Input: part model. Units: mm. Frame: model coordinates. Face numbers are marked on the shaded views. Coordinates: 2 decimals unless noted, no trailing zeros. Loops run counter-clockwise (first coordinate to the right, second up) from the corner with the lowest first, then second, coordinate; pieces in that order, holes last.
```python
from build123d import *

# Parameters (mm, degrees)
F0_R          = 6.3
F0_R_2        = 2.5
F1_DEPTH      = 5
F1_DEPTH_BACK = 6
F6_D          = 2.5
F6_DEPTH      = 5
F6_START      = 0.1252531
F6_TIP        = 0.7510757738


with BuildPart() as f1:
    # F0 (on Front) → F1 (new body, two sides)
    with BuildSketch(Plane.XZ) as f1_sk:
        Circle(F0_R)
        Circle(F0_R_2, mode=Mode.SUBTRACT)
    extrude(amount=-F1_DEPTH)
    extrude(f1_sk.sketch, amount=F1_DEPTH_BACK)

    # F2 (on Right) → F3 (revolve, cut)
    with BuildSketch(Plane.YZ):
        with BuildLine():
            ThreePointArc((0, 6.3), (-2.5, 8.8), (-5, 6.3))
            Line((-5, 6.3), (0, 6.3))
        make_face()
        with BuildLine():
            Line((0, 6.3), (-5, 6.3))
            ThreePointArc((-5, 6.3), (-2.5, 3.8), (0, 6.3))
        make_face()
    revolve(axis=Axis((0, -6, 0), (0, -1, 0)), mode=Mode.SUBTRACT)

    # F6
    # its depths count from where the whole tool has entered the part; down to there all is cleared
    with Locations(Plane.YZ.offset(6.3).offset(-F6_START)):
        with Locations((2.5, 0)):
            Hole(F6_D / 2, depth=F6_DEPTH)
            with Locations((0, 0, -(F6_DEPTH + F6_TIP / 2))):  # 118° drill point
                Cone(0, F6_D / 2, F6_TIP, mode=Mode.SUBTRACT)


solid = f1.part
```
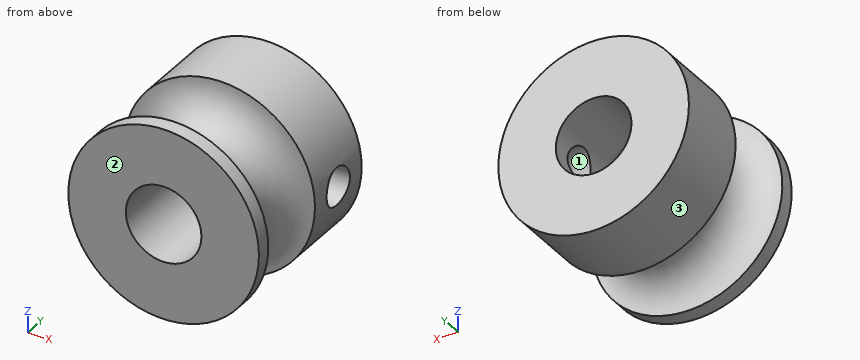
Item 1: Section query A-A (x = 0). Output: boundary loops of the cut face in (y, z), then the cut area to 3 significant figures.
Result:
outline: (-6, -6.3) - (-5, -6.3) arc R2.5 cw to (0, -6.3) - (5, -6.3) - (5, -2.5) - (-6, -2.5) - close; (-6, 2.5) - (5, 2.5) - (5, 6.3) - (0, 6.3) arc R2.5 cw to (-5, 6.3) - (-6, 6.3) - close
area: 64.0 mm2
Item 2: Section query B-B (z = 0). Output: boundary loops of the cut face in (x, y).
Result:
outline: (-6.3, -6) - (-2.5, -6) - (-2.5, 5) - (-6.3, 5) - (-6.3, 0) arc R2.5 cw to (-6.3, -5) - close; (2.5, -6) - (6.3, -6) - (6.3, -5) arc R2.5 cw to (6.3, 0) - (6.3, 1.25) - (2.5, 1.25) - close; (2.5, 3.75) - (6.3, 3.75) - (6.3, 5) - (2.5, 5) - close
Item 3: Section query D-D (x = 5). Count the separate pieces of the cut face and the enclosed holes in it, then the cut area to 3 significant figures.
Result:
separate pieces: 2
enclosed holes: 1
area: 43.9 mm2
Item 4: Mould query, pull axis Z, two halves, no side actions, for the marked faces 1, 2 and 3. Classes: +Z half, -Z half, draft (parallel to the pull), parting line (faces both ways), or undercut.
Result:
face 1: undercut
face 2: draft
face 3: parting line
Item 5: Section query C-C (y = 0.5). Output: boundary loops of the cut face in (x, z).
Result:
outline: circle Ø12.6 at (0, 0); hole circle Ø5 at (0, 0)
Item 6: Contact query for flat-ended pins moving along their axis: P1, Ø1.5, axis at x = 3, y = -1, coming from the +Z side; P2, Ø3, axis at x = 0, z = 0, coming from the -Y side. Output: stop coordinate, or through.
Result:
P1: stops at z = 4.33
P2: passes through
Item 7: Line query: L1, parallel to Z at x = 0, y = 1.25; L2, parallel to Y at x = -2.5, z = 5.75; L3, parallel to Y at x = 4.5, z = 0.75. Output: solid intervals per line, ascending.
Result:
L1: z = -6.3 to -2.5, 2.5 to 6.3
L2: y = -6 to -5, 0 to 5
L3: y = -6 to -4.3, -0.7 to 1.5, 3.5 to 5
